```python
from build123d import *

# Parameters (mm, degrees)
F0_R     = 6.25
F1_DEPTH = 38
F3_DEPTH = 3
F4_R     = 2
F5_DEPTH = 15
F5_TAPER = 3
F6_W     = 8
F6_H     = 15
F7_DEPTH = 10


with BuildPart() as f1:
    # F0 (on Top) → F1 (new body)
    with BuildSketch(Plane.XY):
        Circle(F0_R)
    extrude(amount=F1_DEPTH)

    # F2 (on face) → F3 (join)
    with BuildSketch(Plane.XY.offset(38)):
        with BuildLine():
            ThreePointArc((3.5355339059, -1.25), (3.6959945987, -0.6341324202), (3.75, 0))
            ThreePointArc((3.75, 0), (3.6959945987, 0.6341324202), (3.5355339059, 1.25))
            Line((3.5355339059, 1.25), (-3.5355339059, 1.25))
            ThreePointArc((-3.5355339059, 1.25), (-3.75, 0), (-3.5355339059, -1.25))
            Line((-3.5355339059, -1.25), (3.5355339059, -1.25))
        make_face()
        with BuildLine():
            ThreePointArc((3.5355339059, 1.25), (3.6959945987, 0.6341324202), (3.75, 0))
            ThreePointArc((3.75, 0), (3.6959945987, -0.6341324202), (3.5355339059, -1.25))
            Line((3.5355339059, -1.25), (4.5, -1.25))
            ThreePointArc((4.5, -1.25), (4.8535533906, -1.1035533906), (5, -0.75))
            Line((5, -0.75), (5, 0.75))
            ThreePointArc((5, 0.75), (4.8535533906, 1.1035533906), (4.5, 1.25))
            Line((4.5, 1.25), (3.5355339059, 1.25))
        make_face()
        with BuildLine():
            Line((-3.5355339059, 1.25), (3.5355339059, 1.25))
            ThreePointArc((3.5355339059, 1.25), (0, 3.75), (-3.5355339059, 1.25))
        make_face()
        with BuildLine():
            ThreePointArc((-3.5355339059, -1.25), (0, -3.75), (3.5355339059, -1.25))
            Line((3.5355339059, -1.25), (-3.5355339059, -1.25))
        make_face()
        with BuildLine():
            ThreePointArc((-3.5355339059, -1.25), (-3.75, 0), (-3.5355339059, 1.25))
            Line((-3.5355339059, 1.25), (-4.5, 1.25))
            ThreePointArc((-4.5, 1.25), (-4.8535533906, 1.1035533906), (-5, 0.75))
            Line((-5, 0.75), (-5, -0.75))
            ThreePointArc((-5, -0.75), (-4.8535533906, -1.1035533906), (-4.5, -1.25))
            Line((-4.5, -1.25), (-3.5355339059, -1.25))
        make_face()
    extrude(amount=F3_DEPTH)

    # F4 (on face) → F5 (cut)
    with BuildSketch(Plane.XY.offset(41)):
        Circle(F4_R)
    extrude(amount=-F5_DEPTH, taper=F5_TAPER, mode=Mode.SUBTRACT)

    # F6 (on face) → F7 (cut)
    with BuildSketch(Plane(origin=(0, 0, 0), x_dir=(1, 0, 0), z_dir=(0, 0, -1))):
        with Locations((-6.25, 0)):
            Rectangle(F6_W, F6_H)
    extrude(amount=-F7_DEPTH, mode=Mode.SUBTRACT)


solid = f1.part
```
Read the model definition and answer for the solid it produces. Units are mm, in the model's axes. A direction names the side the tool comes from. Give positions to 0.01 mm unless a question says otherwise; leave off trailing zeros. Loops run counter-clockwise (first coordinate to the right, second up) from the corner with the lowest first, then second, coordinate; pieces in that order, holes last.
Item 1: The mould has two halves that part along X. Classify faces 5 (the flat face through (4, -1.25, 39)), 6 (the conical face through (-0.347, -1.563, 33.395)), 7 (the cylindrical face through (0.06, 3.75, 39.48)): released by +X, released by -X, zero draft, split by the parting line, or undercut.
Item 2: Each of these flat-tipped pins is pushed along its axis until it touches: pin 1 Ø2 at (x, y) = (4, 3.5) entering from +Z; pin 2 Ø5 at (x, z) = (3, 21) entering from +Y; pin 3 Ø0.8 at (x, z) = (-4, 40) entering from -Y. Where does it stop, or does it pass through?
Item 3: For faces 1 (the flat face through (-4, 0, 10)), 2 (the flat face through (4, 1.25, 39)), 3 (the cylindrical face through (-0.06, -3.75, 39.48)), 4 (the flat face through (0, 0, 26)), determine the directions among +Z, -Z, +X, -X, +Y, -Y from which every point of the face is accessible in a straight line to the end or side of a thin tool.
Item 4: The part is cut by section D-D (z = 33). Write down the section's boundary in (x, y), and give its area (3 significant figures).
Item 5: The part is cut by section C-C (y = -4.75). Write down the section's boundary in (x, z).
Item 6: The part is cut by section A-A (x = 0). Write down the section's boundary in (y, z), and give its area (3 significant figures).
Item 7: The part is cut by section B-B (z = 21). Write down the section's boundary in (x, y).
Item 8: Find the intervals of material crossed by line 1 along Z through (x, y) = (-4.75, -0.75); line 2 along Z through (x, y) = (4, -4); line 3 along X through (y, z) = (3.75, 20.5), in increasing order.
Taken from the geometry:
1. face 5: zero draft
1. face 6: undercut
1. face 7: split by the parting line
2. pin 1: stops at z = 38
2. pin 2: stops at y = 6.23
2. pin 3: stops at y = -1.25
3. face 1: -Z, -X, +Y, -Y
3. face 2: +Z, +X, +Y
3. face 3: +Z, -Y
3. face 4: +Z
4. outline: circle Ø12.5 at (0, 0); hole circle Ø3.16 at (0, 0)
4. area: 115 mm2
5. outline: (-4.06, 10) - (-2.25, 10) - (-2.25, 0) - (4.06, 0) - (4.06, 38) - (-4.06, 38) - close
6. outline: (-6.25, 0) - (6.25, 0) - (6.25, 38) - (3.75, 38) - (3.75, 41) - (2, 41) - (1.21, 26) - (-1.21, 26) - (-2, 41) - (-3.75, 41) - (-3.75, 38) - (-6.25, 38) - close
6. area: 449 mm2
7. outline: circle Ø12.5 at (0, 0)
8. line 1: z = 10 to 41
8. line 2: z = 0 to 38
8. line 3: x = -5 to 5
